Geometry: see drawing. Coordinates: mm, zero at the bounding-box minimum. A direction names the side the tool comes from. Coordinates: 2 decimals unless noted, no trailing zeros. Write each loop counter-clockwise with the first axis right and the second up, starting at its lowest first coordinate (ties: lowest second). Pieces come first, ordered by that corner, then holes.
1) Section query B-B (y = 23.5). Output: boundary loops of the cut face in (x, z) (1 decimal), then the cut area to 3 significant figures.
2) Section query A-A (x = 18.5). Output: boundary loops of the cut face in (y, z), then the cut area to 3 significant figures.
3) Section query D-D (y = 29.5). Output: boundary loops of the cut face in (x, z), then the cut area to 3 significant figures.
4) Line query: L1, parallel to Z at x = 8.5, y = 29.5; L2, parallel to Z at x = 15, y = 27.5; L3, parallel to Y at x = 34.25, z = 56.25 (1 decimal). Output: solid intervals per line, ascending.
5) Set-up query: the marked faces 1, 2 and 3. Return all of +Z, -Z, +X, -X, +Y, -Y with unobstructed straight access to the full face (end or side cutting, diameter ignored); none if empty.
6) Pin query (flat end, axial travel): pin 1 Ø2.5 at (x, y) = (2, 18.5) entering from +Z; pin 2 Ø8 at (x, z) = (26, 45.5) entering from -Y; pin 3 Ø6 at (x, y) = (31, 29) entering from -Z; pin 4 Ø0.9 at (x, y) = (26, 4) entering from +Z. Return the tip coordinate at first contact, or that it passes through.
7) Section query C-C (z = 20). Output: boundary loops of the cut face in (x, y), then the cut area to 3 significant figures.
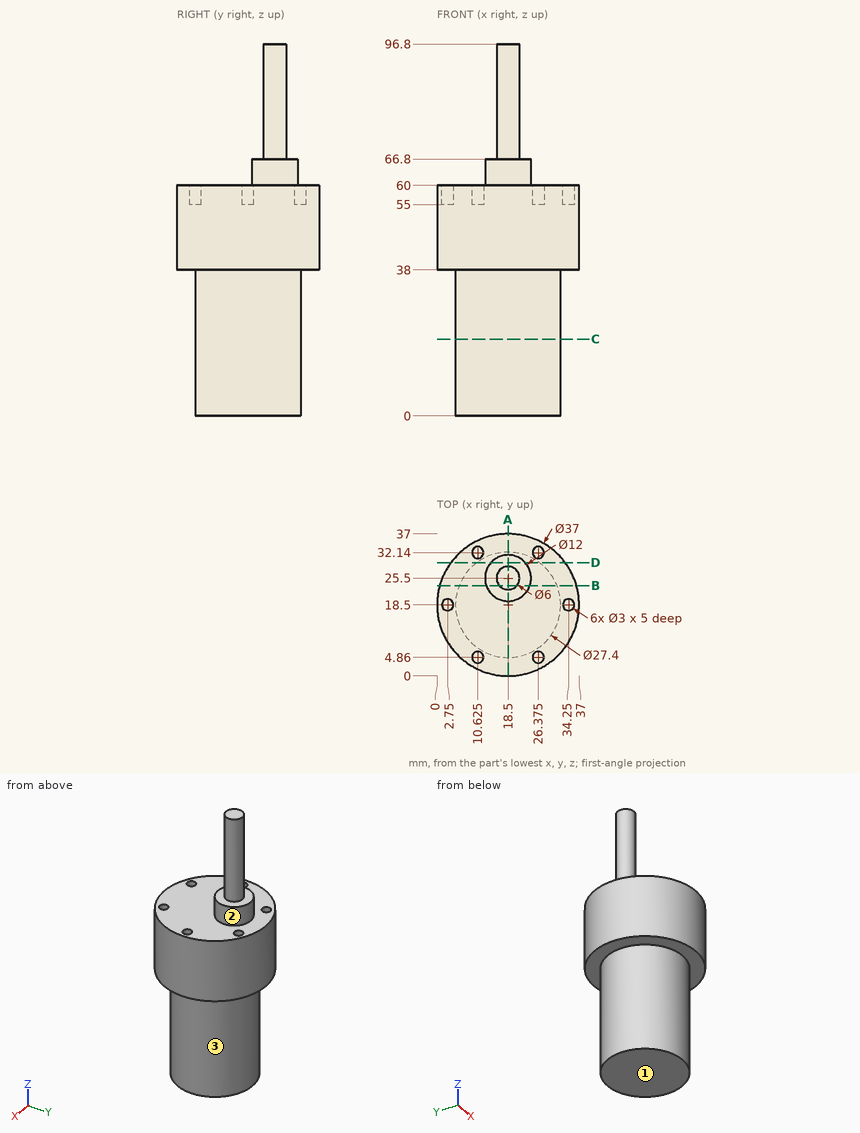
Answer:
1. outline: (0.7, 38) - (5.7, 38) - (5.7, 0) - (31.3, 0) - (31.3, 38) - (36.3, 38) - (36.3, 60) - (24.2, 60) - (24.2, 66.8) - (20.7, 66.8) - (20.7, 96.8) - (16.3, 96.8) - (16.3, 66.8) - (12.8, 66.8) - (12.8, 60) - (0.7, 60) - close
1. area: 1,960 mm2
2. outline: (0, 38) - (4.8, 38) - (4.8, 0) - (32.2, 0) - (32.2, 38) - (37, 38) - (37, 60) - (31.5, 60) - (31.5, 66.8) - (28.5, 66.8) - (28.5, 96.8) - (22.5, 96.8) - (22.5, 66.8) - (19.5, 66.8) - (19.5, 60) - (0, 60) - close
2. area: 2,120 mm2
3. outline: (3.63, 38) - (10.33, 38) - (10.33, 0) - (26.67, 0) - (26.67, 38) - (33.37, 38) - (33.37, 60) - (22.97, 60) - (22.97, 66.8) - (14.03, 66.8) - (14.03, 60) - (3.63, 60) - close
3. area: 1,340 mm2
4. L1: z = 38 to 60
4. L2: z = 0 to 66.8
4. L3: y = 8.8 to 17, 20 to 28.2
5. face 1: -Z, +X, -X, +Y, -Y
5. face 2: +Z
5. face 3: -Z
6. pin 1: stops at z = 60
6. pin 2: stops at y = 0.33
6. pin 3: stops at z = 0
6. pin 4: stops at z = 55
7. outline: circle Ø27.4 at (18.5, 18.5)
7. area: 590 mm2
